Input: part model. Units: mm. Frame: model coordinates. Face numbers are marked on the shaded views. A direction names the side the tool comes from. Give positions to 0.01 mm unless a question says otherwise; leave off trailing zeros. Write each loop counter-clockwise with the first axis right and the second up, starting at its lowest first coordinate (ties: lowest second). Pieces come first, ordered by that corner, then holes. Notation, with made-up numbers: (65, 32.25) - (78, 32.25) arc R10 ccw to (78, 50.25) - close; hole circle Ø11 at (31.25, 55.25). An arc over 180 degrees is marked (long way). Answer as CSV lines item,"result".
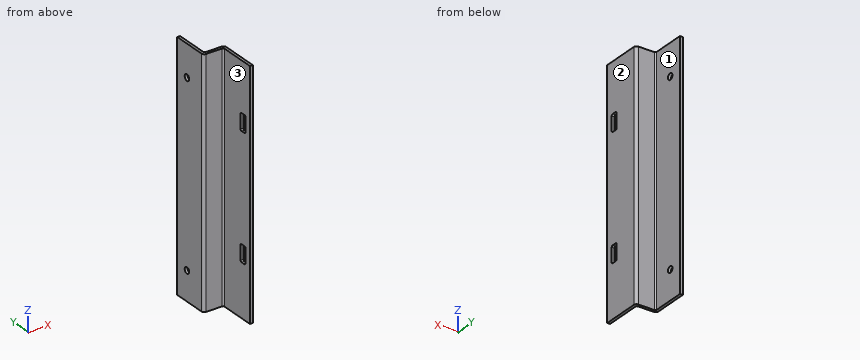
```python
from build123d import *

# Parameters (mm, degrees)
F1_DEPTH = 228
F2_R     = 3
F3_DEPTH = 2.7
F5_DEPTH = 2.7


with BuildPart() as f1:
    # F0 (on Top) → F1 (new body)
    with BuildSketch(Plane.XY):
        with BuildLine():
            Line((2.7, 0), (0, 0))
            Line((0, 0), (0, -32.5))
            ThreePointArc((0, -32.5), (0.732233, -34.267767), (2.5, -35))
            Line((2.5, -35), (17.75, -35))
            ThreePointArc((17.75, -35), (18.633883, -35.366117), (19, -36.25))
            Line((19, -36.25), (19, -70.3))
            Line((19, -70.3), (21.7, -70.3))
            Line((21.7, -70.3), (21.7, -34.8))
            ThreePointArc((21.7, -34.8), (20.967767, -33.032233), (19.2, -32.3))
            Line((19.2, -32.3), (3.95, -32.3))
            ThreePointArc((3.95, -32.3), (3.066117, -31.933883), (2.7, -31.05))
            Line((2.7, -31.05), (2.7, 0))
        make_face()
    extrude(amount=F1_DEPTH)

    # F2 (on face) → F3 (cut)
    with BuildSketch(Plane(origin=(0, 0, 0), x_dir=(0, -1, 0), z_dir=(-1, 0, 0))):
        with Locations((13, 198)):
            Circle(F2_R)
        with Locations((13, 27.5)):
            Circle(F2_R)
    extrude(amount=-F3_DEPTH, mode=Mode.SUBTRACT)

    # F4 (on face) → F5 (cut)
    with BuildSketch(Plane.YZ.offset(21.7)):
        with BuildLine():
            ThreePointArc((-57.8, 64.25), (-58.166117, 65.133883), (-59.05, 65.5))
            Line((-59.05, 65.5), (-63.05, 65.5))
            ThreePointArc((-63.05, 65.5), (-63.933883, 65.133883), (-64.3, 64.25))
            Line((-64.3, 64.25), (-64.3, 50.75))
            ThreePointArc((-64.3, 50.75), (-63.933883, 49.866117), (-63.05, 49.5))
            Line((-63.05, 49.5), (-59.05, 49.5))
            ThreePointArc((-59.05, 49.5), (-58.166117, 49.866117), (-57.8, 50.75))
            Line((-57.8, 50.75), (-57.8, 64.25))
        make_face()
        with BuildLine():
            ThreePointArc((-57.8, 180.25), (-58.166117, 181.133883), (-59.05, 181.5))
            Line((-59.05, 181.5), (-63.05, 181.5))
            ThreePointArc((-63.05, 181.5), (-63.933883, 181.133883), (-64.3, 180.25))
            Line((-64.3, 180.25), (-64.3, 166.75))
            ThreePointArc((-64.3, 166.75), (-63.933883, 165.866117), (-63.05, 165.5))
            Line((-63.05, 165.5), (-59.05, 165.5))
            ThreePointArc((-59.05, 165.5), (-58.166117, 165.866117), (-57.8, 166.75))
            Line((-57.8, 166.75), (-57.8, 180.25))
        make_face()
    extrude(amount=-F5_DEPTH, mode=Mode.SUBTRACT)


solid = f1.part
```
Item 1: Cut plane D-D on x = 9.5. Return the cut outline in (y, z), plus the area to 3 significant figures.
The answers:
outline,"(-35, 0) - (-32.3, 0) - (-32.3, 228) - (-35, 228) - close"
area,"616 mm²"
Item 2: Cut plane B-B on y = -13. Return the cut outline in (x, z).
The answers:
outline,"(0, 0) - (2.7, 0) - (2.7, 24.5) - (0, 24.5) - close; (0, 30.5) - (2.7, 30.5) - (2.7, 195) - (0, 195) - close; (0, 201) - (2.7, 201) - (2.7, 228) - (0, 228) - close"
Item 3: Cut plane A-A on z = 198. Return the cut outline in (x, y), plus the area to 3 significant figures.
The answers:
outline,"(0, -32.5) arc R2.5 ccw to (2.5, -35) - (17.75, -35) arc R1.25 cw to (19, -36.25) - (19, -70.3) - (21.7, -70.3) - (21.7, -34.8) arc R2.5 ccw to (19.2, -32.3) - (3.95, -32.3) arc R1.25 cw to (2.7, -31.05) - (2.7, -16) - (0, -16) - close; (0, -10) - (2.7, -10) - (2.7, 0) - (0, 0) - close"
area,"223 mm²"
Item 4: Reachability of the marked faces 1, 2 and 3 from +Z, -Z, +X, -X, +Y, -Y: full face, straight path, thin tool, end or side. Return the list, or none.
The answers:
face 1,"+Z, -Z, +X, +Y"
face 2,"+Z, -Z, +X, +Y, -Y"
face 3,"+Z, -Z, -X, -Y"
Item 5: Ray query, line 1 (Z direction, x = 2, y = -13); line 2 (Y direction, x = 12, z = 53); line 3 (X direction, y = -54.5, z = 27). Return the intervals inside material, ascending. Write a range as from..to.
The answers:
line 1,"0..24.5, 30.5..195, 201..228"
line 2,"-35..-32.3"
line 3,"19..21.7"
Item 6: Contact query for flat-ended pins moving along their axis: pin 1 (1.5 mm diameter, centred on y = -32, z = 150.5, fed in from +X); pin 2 (2 mm diameter, centred on x = 8.5, z = 196, fed in from +Y); pin 3 (2 mm diameter, centred on y = -30, z = 90, fed in from +X). Output: stop coordinate, or through.
The answers:
pin 1,"x = 20.63"
pin 2,"y = -32.3"
pin 3,"x = 2.7"
Item 7: Cut plane C-C on z = 155. Return the cut outline in (x, y), plus the area to 3 significant figures.
The answers:
outline,"(0, -32.5) arc R2.5 ccw to (2.5, -35) - (17.75, -35) arc R1.25 cw to (19, -36.25) - (19, -70.3) - (21.7, -70.3) - (21.7, -34.8) arc R2.5 ccw to (19.2, -32.3) - (3.95, -32.3) arc R1.25 cw to (2.7, -31.05) - (2.7, 0) - (0, 0) - close"
area,"239 mm²"
